Can you work these out from the model? Positions are in its coordinate system, mm. Give positions to 0.01 mm unless a question says otherwise; leave off trailing zeros. Order: outer loops, then holes, each group sorted by start corner. A loop starts at its lowest first (then second) coordinate and runs counter-clockwise, first axis right, second up. Notation, with made-up numbers: (28.5, -11) - (60.5, -11) arc R30 ccw to (60.5, 12) - close; hole circle Ø6 at (-12, 85.25). An arc over 180 degrees is marked (long way). Answer as a JSON object with one key per item and string values.
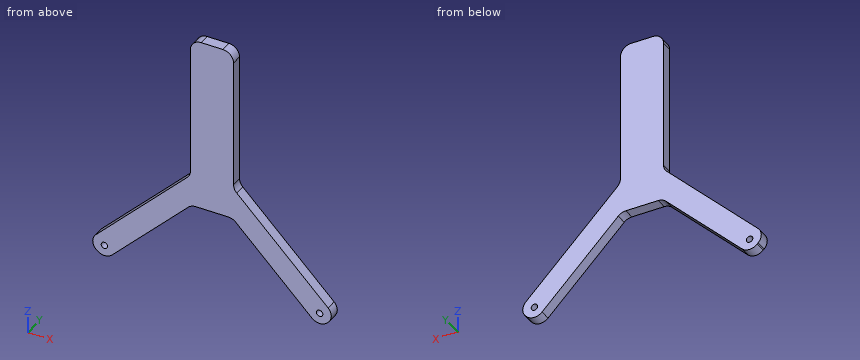
```python
from build123d import *

# Parameters (mm, degrees)
SKETCH1_R           = 3.81
BOSS_EXTRUDE1_DEPTH = 12.7


with BuildPart() as part:
    # Sketch1 → Boss-Extrude1 (new body)
    with BuildSketch(Plane(origin=(0, 0, 0), x_dir=(1, 0, 0), z_dir=(0, 1, 0))):
        with BuildLine():
            Line((-3.719743879, 3.719743879), (-111.482817332, 111.482817332))
            ThreePointArc((-111.482817332, 111.482817332), (-115.202561211, 120.463073453), (-111.482817332, 129.443329574))
            Line((-111.482817332, 129.443329574), (-110.393329574, 130.532817332))
            ThreePointArc((-110.393329574, 130.532817332), (-101.413073453, 134.252561211), (-92.432817332, 130.532817332))
            Line((-92.432817332, 130.532817332), (-2.630256121, 40.730256121))
            ThreePointArc((-2.630256121, 40.730256121), (1.489920409, 37.977242179), (6.35, 37.010512242))
            Line((6.35, 37.010512242), (44.45, 37.010512242))
            ThreePointArc((44.45, 37.010512242), (49.310079591, 37.977242179), (53.430256121, 40.730256121))
            Line((53.430256121, 40.730256121), (143.232817332, 130.532817332))
            ThreePointArc((143.232817332, 130.532817332), (152.213073453, 134.252561211), (161.193329574, 130.532817332))
            Line((161.193329574, 130.532817332), (162.282817332, 129.443329574))
            ThreePointArc((162.282817332, 129.443329574), (166.002561211, 120.463073453), (162.282817332, 111.482817332))
            Line((162.282817332, 111.482817332), (54.519743879, 3.719743879))
            ThreePointArc((54.519743879, 3.719743879), (51.766729937, -0.400432651), (50.8, -5.260512242))
            Line((50.8, -5.260512242), (50.8, -157.660512242))
            ThreePointArc((50.8, -157.660512242), (47.080256121, -166.640768363), (38.1, -170.360512242))
            Line((38.1, -170.360512242), (12.7, -170.360512242))
            ThreePointArc((12.7, -170.360512242), (3.719743879, -166.640768363), (0, -157.660512242))
            Line((0, -157.660512242), (0, -5.260512242))
            ThreePointArc((0, -5.260512242), (-0.966729937, -0.400432651), (-3.719743879, 3.719743879))
        make_face()
        with Locations(Location((152.213073453, 121.552561211, 0), (0, 0, 270))):
            Circle(SKETCH1_R, mode=Mode.SUBTRACT)
        with Locations(Location((-101.413073453, 121.552561211, 0), (0, 0, 270))):
            Circle(SKETCH1_R, mode=Mode.SUBTRACT)
    extrude(amount=BOSS_EXTRUDE1_DEPTH)


solid = part.part
```
Q1. If we section it at C-C, the plane x = 133: Please give me the cut outline in (y, z), then the cut area to 3 significant figures.
Recorded:
{"outline": "(0, -120.3) - (12.7, -120.3) - (12.7, -82.2) - (0, -82.2) - close", "area": "484 mm^2"}
Q2. If we section it at D-D, the plane z = 56.5: Please give me the cut outline in (x, y).
Recorded:
{"outline": "(0, 0) - (50.8, 0) - (50.8, 12.7) - (0, 12.7) - close"}
Q3. If we section it at B-B, the plane y = 3: Please give me the cut outline in (x, z).
Recorded:
{"outline": "(-111.48, -129.44) - (-110.39, -130.53) arc R12.7 ccw to (-92.43, -130.53) - (-2.63, -40.73) arc R12.7 cw to (6.35, -37.01) - (44.45, -37.01) arc R12.7 cw to (53.43, -40.73) - (143.23, -130.53) arc R12.7 ccw to (161.19, -130.53) - (162.28, -129.44) arc R12.7 ccw to (162.28, -111.48) - (54.52, -3.72) arc R12.7 cw to (50.8, 5.26) - (50.8, 157.66) arc R12.7 ccw to (38.1, 170.36) - (12.7, 170.36) arc R12.7 ccw to (0, 157.66) - (0, 5.26) arc R12.7 cw to (-3.72, -3.72) - (-111.48, -111.48) arc R12.7 ccw to start; hole circle Ø7.62 at (-101.41, -121.55); hole circle Ø7.62 at (152.21, -121.55)"}
Q4. If we section it at A-A, the plane z = -97: Please give me the cut outline in (x, y), then the cut area to 3 significant figures.
Recorded:
{"outline": "(-97, 0) - (-58.9, 0) - (-58.9, 12.7) - (-97, 12.7) - close; (109.7, 0) - (147.8, 0) - (147.8, 12.7) - (109.7, 12.7) - close", "area": "968 mm^2"}
Q5. I'm going to push flat-ended pins straight in: pin 1 Ø3 at (x, y) = (111, 2) entering from -Z; pin 2 Ø4 at (x, y) = (133, 5) entering from +Z; pin 3 Ø2 at (y, z) = (1.5, -60) entering from +X. Where does each tip first touch, or does it pass through?
Recorded:
{"pin 1": "stops at z = -99.8", "pin 2": "stops at z = -80.2", "pin 3": "stops at x = 111.8"}
Q6. I need wall thicknesses on L1, parallel to X at y = 11.75, z = -119; L2, parallel to X at y = 4, z = 100; L3, parallel to X at y = 10.5, z = -53. Which ranges of each line are inside material? Lowest first, please.
Recorded:
{"L1": "x = -115.12 to -104.24, -98.58 to -80.9, 131.7 to 149.38, 155.04 to 165.92", "L2": "x = 0 to 50.8", "L3": "x = -53 to -14.9, 65.7 to 103.8"}
